Work out the finished part from the listing and answer in its coordinate system (mm). A direction names the side the tool comes from. Coordinates: 2 decimals unless noted, no trailing zeros. Write each loop counter-clockwise with the first axis right and the second up, starting at its lowest first coordinate (ties: lowest second). Pieces come first, ordered by that corner, then holes. Notation, with made-up numbers: (-38, -8) - (-17, -8) arc R34 ccw to (-17, 29) - close; hole circle Ø6 at (-34.75, 21). An arc over 180 degrees is marked (long way). Use CSV: the item, a comma, the result in double quotes. Start each with the question number.
from build123d import *

# Parameters (mm, degrees)
CROQUIS2_R            = 3.05
CORTAR_EXTRUIR1_DEPTH = 10


with BuildPart() as part:
    # Croquis1 → Revolución1 (revolve)
    with BuildSketch(Plane.XY, mode=Mode.PRIVATE) as revoluci_n1_sk:
        Polygon((0, 8.266073618), (8, 8.266073618), (8, -3.733926382), (6, -3.733926382), (4.5, -15.733926382), (0, -15.733926382), align=None)
    revolve(revoluci_n1_sk.sketch.rotate(Axis((0, 12.501582414, 0), (0, -1, 0)), 180), axis=Axis((0, 12.501582414, 0), (0, -1, 0)))

    # Croquis2 → Cortar-Extruir1 (cut)
    with BuildSketch(Plane(origin=(0, 8.266073618, 0), x_dir=(1, 0, 0), z_dir=(0, 1, 0))):
        with Locations(Location((0, 0, 0), (0, 0, 180))):
            Circle(CROQUIS2_R)
    extrude(amount=-CORTAR_EXTRUIR1_DEPTH, mode=Mode.SUBTRACT)


solid = part.part
Item 1: A cutting plane is placed at C-C (y = 0). Determine the outline of the cut face in (x, z), then the cut area to 3 significant figures.
Item 2: A cutting plane is placed at B-B (x = 0). Determine the outline of the cut face in (y, z).
Item 3: A cutting plane is placed at A-A (z = 0). Determine the outline of the cut face in (x, y), then the cut area to 3 significant figures.
Item 4: Each of these flat-tipped pins is pushed along its axis until it touches: pin 1 (1.5 mm diameter, centred on y = -10, z = 5, fed in from -X); pin 2 (6.5 mm diameter, centred on x = -1, z = 0, fed in from +Y); pin 3 (5 mm diameter, centred on x = 3.5, y = -8, fed in from -Z); pin 4 (2 mm diameter, centred on y = -7.5, z = -3.5, fed in from -X). Where does it stop, or does it pass through?
Item 5: Which of the six approach directions +Z, -Z, +X, -X, +Y, -Y give full straight-line access (tool end or side, diameter ignored) to faces 1 (the face through (0, -1.734, 0)), 2 (the face through (3.4, 8.266, -0.1))?
Item 6: Determine the mould class of faces 3 (the face through (4.158, -9.818, 3.188)), 4 (the face through (2, -3.734, -6)), 5 (the face through (3.047, 3.336, 0.134)) for opening direction X: +X half, -X half, draft (parallel to the pull), parting line (faces both ways), or undercut.
Item 7: A cutting plane is placed at D-D (y = -12.5). Determine the outline of the cut face in (x, z).
Item 8: Straight lines are drawn through the part: probe 1 along Z at (x, y) = (0, 2.25); probe 2 along Y at (x, z) = (6.25, 3.5); probe 3 along Z at (x, y) = (5, -4.5). For each, find the intervals that lie inside material, in ascending order. Write a range as [from, to].
Calculated:
1,outline,"circle Ø16 at (0, 0); hole circle Ø6.1 at (0, 0)"
1,area,"172 mm²"
2,outline,"(-15.73, -4.5) - (-3.73, -6) - (-3.73, -8) - (8.27, -8) - (8.27, -3.05) - (-1.73, -3.05) - (-1.73, 3.05) - (8.27, 3.05) - (8.27, 8) - (-3.73, 8) - (-3.73, 6) - (-15.73, 4.5) - close"
3,outline,"(-8, -3.73) - (-6, -3.73) - (-4.5, -15.73) - (4.5, -15.73) - (6, -3.73) - (8, -3.73) - (8, 8.27) - (3.05, 8.27) - (3.05, -1.73) - (-3.05, -1.73) - (-3.05, 8.27) - (-8, 8.27) - close"
3,area,"257 mm²"
4,pin 1,"stops at x = -3.04"
4,pin 2,"stops at y = 8.27"
4,pin 3,"stops at z = -5.46"
4,pin 4,"stops at x = -4.95"
5,face 1,"+Y"
5,face 2,"+Z, -Z, +X, -X, +Y"
6,face 3,"parting line"
6,face 4,"draft"
6,face 5,"undercut"
7,outline,"circle Ø9.81 at (0, 0)"
8,probe 1,"z = [-8, -3.05], [3.05, 8]"
8,probe 2,"y = [-3.73, 8.27]"
8,probe 3,"z = [-3.14, 3.14]"
